```python
from build123d import *

# Parameters (mm, degrees)
BOSS_EXTRUDE1_DEPTH = 1.6
BOSS_EXTRUDE2_DEPTH = 8.5
BOSS_EXTRUDE3_DEPTH = 9
SKETCH4_R           = 1.1
CUT_EXTRUDE1_DEPTH  = 64.607734681


with BuildPart() as part:
    # Sketch1 → Boss-Extrude1 (new body)
    with BuildSketch(Plane(origin=(0, 0, 0), x_dir=(1, 0, 0), z_dir=(0, 1, 0))):
        with BuildLine():
            Line((-11.77766953, 17.67766953), (-11.77766953, 31))
            Line((-11.77766953, 31), (11.77766953, 31))
            Line((11.77766953, 31), (11.77766953, 17.67766953))
            ThreePointArc((11.77766953, 17.67766953), (13.505739521, 13.505739521), (17.67766953, 11.77766953))
            Line((17.67766953, 11.77766953), (33.07278358, 11.77766953))
            ThreePointArc((33.07278358, 11.77766953), (35.1073, 0), (33.07278358, -11.77766953))
            Line((33.07278358, -11.77766953), (17.67766953, -11.77766953))
            ThreePointArc((17.67766953, -11.77766953), (11.77766953, -17.67766953), (17.67766953, -23.57766953))
            Line((17.67766953, -23.57766953), (30.09766953, -23.57766953))
            Line((30.09766953, -23.57766953), (36.017643771, -30.655106364))
            ThreePointArc((36.017643771, -30.655106364), (0, -47.297), (-36.017643771, -30.655106364))
            Line((-36.017643771, -30.655106364), (-30.09766953, -23.57766953))
            Line((-30.09766953, -23.57766953), (-17.67766953, -23.57766953))
            ThreePointArc((-17.67766953, -23.57766953), (-11.77766953, -17.67766953), (-17.67766953, -11.77766953))
            Line((-17.67766953, -11.77766953), (-26, -11.77766953))
            Line((-26, -11.77766953), (-26, 11.77766953))
            Line((-26, 11.77766953), (-17.67766953, 11.77766953))
            ThreePointArc((-17.67766953, 11.77766953), (-13.505739521, 13.505739521), (-11.77766953, 17.67766953))
        make_face()
    extrude(amount=BOSS_EXTRUDE1_DEPTH)

    # Sketch2 → Boss-Extrude2 (add)
    with BuildSketch(Plane(origin=(0, 1.6, 0), x_dir=(1, 0, 0), z_dir=(0, 1, 0))):
        Polygon((-33.597062742, -27.864051564), (-23.868298315, -36.027454207), (-20.602937258, -32.135948436), (-30.331701685, -23.972545793), align=None)
        Polygon((23.868298315, -36.027454207), (33.597062742, -27.864051564), (30.331701685, -23.972545793), (20.602937258, -32.135948436), align=None)
    extrude(amount=BOSS_EXTRUDE2_DEPTH)

    # Sketch3 → Boss-Extrude3 (add)
    with BuildSketch(Plane(origin=(0, 1.6, 0), x_dir=(1, 0, 0), z_dir=(0, 1, 0))):
        Polygon((-25.517948101, -44.939697826), (-19.990220336, -32.623276846), (-10.866945536, -36.717890005), (-16.394673301, -49.034310985), align=None)
        Polygon((-0.36916096, -38.28278004), (-2.261296496, -51.649523215), (-12.162587737, -50.247941336), (-10.2704522, -36.881198161), align=None)
        Polygon((2.261296496, -51.649523215), (0.36916096, -38.28278004), (10.2704522, -36.881198161), (12.162587737, -50.247941336), align=None)
        Polygon((16.394673301, -49.034310985), (10.866945536, -36.717890005), (19.990220336, -32.623276846), (25.517948101, -44.939697826), align=None)
    extrude(amount=BOSS_EXTRUDE3_DEPTH)

    # Sketch4 → Cut-Extrude1 (cut, through all)
    with BuildSketch(Plane(origin=(0, 1.6, 0), x_dir=(1, 0, 0), z_dir=(0, 1, 0))):
        with Locations(Location((0, -34.8, 0), (0, 0, 270))):
            Circle(SKETCH4_R)
        with Locations(Location((25, 0, 0), (0, 0, 270))):
            Circle(SKETCH4_R)
        with Locations(Location((-23, 0, 0), (0, 0, 270))):
            Circle(SKETCH4_R)
        with Locations(Location((-9, 28, 0), (0, 0, 270))):
            Circle(SKETCH4_R)
        with Locations(Location((9, 28, 0), (0, 0, 270))):
            Circle(SKETCH4_R)
    extrude(amount=-CUT_EXTRUDE1_DEPTH, mode=Mode.SUBTRACT)


solid = part.part
```
Input: part model. Units: mm. Frame: model coordinates. A direction names the side the tool comes from. Give positions to 0.01 mm unless a question says otherwise; leave off trailing zeros. Write each loop counter-clockwise with the first axis right and the second up, starting at its lowest first coordinate (ties: lowest second). Pieces come first, ordered by that corner, then holes. Notation, with made-up numbers: (-40, 63) - (-1, 63) arc R6 ccw to (-1, 67) - close; hole circle Ø10 at (2, 63.5). An arc over 180 degrees is marked (long way). Write item = value, one per line. Start each with the question number.
1. First-contact query: pin 1 Ø5 at (x, y) = (16, 8) entering from +Z; pin 2 Ø0.5 at (x, y) = (-22, 0.5) entering from +Z; pin 3 Ø6 at (x, y) = (25.5, 2) entering from -Z. Flat tips, straight axial feed; report the tip coordinate or a pass-through.
2. Section query D-D, the plane x = 27. Output: boundary loops of the cut face in (y, z), then the cut area to 3 significant figures.
3. Section query A-A, the plane z = 0. Output: boundary loops of the cut face in (x, y).
4. Section query C-C, the plane z = 35. Output: boundary loops of the cut face in (x, y).
5. Access query for faces 4 (the flat face through (-31.94, 5.79, 25.89)), 5 (the flat face through (31.99, 5.79, 25.95)), 6 (the cylindrical face through (0.573, 0.789, 47.294)), 7 (the flat face through (11.203, 6.037, 43.471)). Directions: +Z, -Z, +X, -X, +Y, -Y. A direction counts if a zero-diameter tool reaches every point of the face in a straight line with its end or side. Return the directions, or none.
6. Section query B-B, the plane y = 5.25. Output: boundary loops of the cut face in (x, z), then the cut area to 3 significant figures.
7. Ray query, L1, parallel to X at y = 0.6, z = -28; L2, parallel to Y at x = 28, z = 28; L3, parallel to X at y = 1.15, z = 34.8. Return the intervals inside material, ascending.
8. Mould query, pull axis X, two halves, no side actions, for faces 1 (the flat face through (-7.14, 6.04, 50.96)), 2 (the flat face through (-22.26, 5.79, 34.11)), 3 (the flat face through (-20, 1.6, 45)). Classes: released by +X, released by -X, zero draft, split by the parting line, or undercut.
Check sheet entries:
q1.pin_1 = 49.03
q1.pin_2 = 42
q1.pin_3 = -11.78
q2.outline = (0, -11.78) - (1.6, -11.78) - (1.6, 11.78) - (0, 11.78) - close; (0, 23.58) - (1.6, 23.58) - (1.6, 26.77) - (10.1, 26.77) - (10.1, 33.4) - (1.6, 33.4) - (1.6, 38.83) - (0, 38.83) - close
q2.area = 118 mm2
q3.outline = (-26, 0) - (-24.1, 0) - (-24.1, 1.6) - (-26, 1.6) - close; (-21.9, 0) - (23.9, 0) - (23.9, 1.6) - (-21.9, 1.6) - close; (26.1, 0) - (35.11, 0) - (35.11, 1.6) - (26.1, 1.6) - close
q4.outline = (-31.81, 0) - (-1.08, 0) - (-1.08, 1.6) - (-14.69, 1.6) - (-14.69, 10.6) - (-21.06, 10.6) - (-21.06, 1.6) - (-23.01, 1.6) - (-23.01, 10.1) - (-25.09, 10.1) - (-25.09, 1.6) - (-31.81, 1.6) - close; (1.08, 0) - (31.81, 0) - (31.81, 1.6) - (25.09, 1.6) - (25.09, 10.1) - (23.01, 10.1) - (23.01, 1.6) - (21.06, 1.6) - (21.06, 10.6) - (14.69, 10.6) - (14.69, 1.6) - (1.08, 1.6) - close
q5.face_4 = -Z, -X, +Y
q5.face_5 = -Z, +X, +Y
q5.face_6 = +Z, -Y
q5.face_7 = +Y
q6.outline = (-33.6, 27.86) - (-30.33, 23.97) - (-20.6, 32.14) - (-23.87, 36.03) - close; (-25.52, 44.94) - (-19.99, 32.62) - (-10.87, 36.72) - (-16.39, 49.03) - close; (-12.16, 50.25) - (-10.27, 36.88) - (-0.37, 38.28) - (-2.26, 51.65) - close; (0.37, 38.28) - (10.27, 36.88) - (12.16, 50.25) - (2.26, 51.65) - close; (10.87, 36.72) - (19.99, 32.62) - (25.52, 44.94) - (16.39, 49.03) - close; (20.6, 32.14) - (30.33, 23.97) - (33.6, 27.86) - (23.87, 36.03) - close
q6.area = 669 mm2
q7.L1 = -11.78 to -10.1, -7.9 to 7.9, 10.1 to 11.78
q7.L2 = 0 to 10.1
q7.L3 = -32.03 to -1.1, 1.1 to 32.03
q8.face_1 = released by -X
q8.face_2 = undercut
q8.face_3 = zero draft
